from build123d import *

# Parameters (mm, degrees)
BOSS_EXTRUDE1_DEPTH = 25
CUT_EXTRUDE1_DEPTH  = 23
BOSS_EXTRUDE2_DEPTH = 25
BOSS_EXTRUDE3_DEPTH = 2
SKETCH6_R           = 4
BOSS_EXTRUDE4_DEPTH = 10
SKETCH7_R           = 2
CUT_EXTRUDE2_DEPTH  = 54
SKETCH8_R           = 3.5
CUT_EXTRUDE3_DEPTH  = 10
BOSS_EXTRUDE5_DEPTH = 1
FILLET1_R           = 1
SKETCH11_W          = 25
SKETCH11_H          = 84.5
BOSS_EXTRUDE7_DEPTH = 22
CUT_EXTRUDE4_DEPTH  = 34.548411539
SKETCH13_W          = 8.2
SKETCH13_H          = 0.499092091
CUT_EXTRUDE5_DEPTH  = 94.548411539
SKETCH14_W          = 54
SKETCH14_H          = 88
SKETCH14_W_2        = 48
SKETCH14_H_2        = 82.5
CUT_EXTRUDE6_DEPTH  = 1
CUT_EXTRUDE7_DEPTH  = 2
SKETCH16_W          = 8
SKETCH16_H          = 6
CUT_EXTRUDE9_DEPTH  = 2
SKETCH17_W          = 18
SKETCH17_H          = 32
BOSS_EXTRUDE8_DEPTH = 4
SKETCH18_W          = 1.390332564
SKETCH18_H          = 32
BOSS_EXTRUDE9_DEPTH = 3
SKETCH19_W          = 9
SKETCH19_H          = 3.2
CUT_EXTRUDE10_DEPTH = 6
FILLET2_R           = 1
FILLET3_R           = 1
FILLET4_R           = 1
FILLET5_R           = 1
CUT_EXTRUDE12_DEPTH = 1


with BuildPart() as part:
    # Sketch1 → Boss-Extrude1 (new body)
    with BuildSketch(Plane(origin=(0, 0, 0), x_dir=(1, 0, 0), z_dir=(0, 1, 0))):
        with BuildLine():
            Line((-80, 62), (80, 62))
            ThreePointArc((80, 62), (101.213203436, 53.213203436), (110, 32))
            Line((110, 32), (110, -32))
            ThreePointArc((110, -32), (101.213203436, -53.213203436), (80, -62))
            Line((80, -62), (-80, -62))
            ThreePointArc((-80, -62), (-101.213203436, -53.213203436), (-110, -32))
            Line((-110, -32), (-110, 32))
            ThreePointArc((-110, 32), (-101.213203436, 53.213203436), (-80, 62))
        make_face()
    extrude(amount=BOSS_EXTRUDE1_DEPTH)

    # Sketch2 → Cut-Extrude1 (cut)
    with BuildSketch(Plane(origin=(0, 25, 0), x_dir=(1, 0, 0), z_dir=(0, 1, 0))):
        with BuildLine():
            Line((-80, -60), (80, -60))
            ThreePointArc((80, -60), (99.798989873, -51.798989873), (108, -32))
            Line((108, -32), (108, 32))
            ThreePointArc((108, 32), (99.798989873, 51.798989873), (80, 60))
            Line((80, 60), (-80, 60))
            ThreePointArc((-80, 60), (-99.798989873, 51.798989873), (-108, 32))
            Line((-108, 32), (-108, -32))
            ThreePointArc((-108, -32), (-99.798989873, -51.798989873), (-80, -60))
        make_face()
    extrude(amount=-CUT_EXTRUDE1_DEPTH, mode=Mode.SUBTRACT)

    # Sketch3 → Boss-Extrude2 (add)
    with BuildSketch(Plane(origin=(0, 2, 0), x_dir=(1, 0, 0), z_dir=(0, 1, 0))):
        with BuildLine():
            Line((-80, -60), (80, -60))
            ThreePointArc((80, -60), (99.798989873, -51.798989873), (108, -32))
            Line((108, -32), (108, 32))
            ThreePointArc((108, 32), (99.798989873, 51.798989873), (80, 60))
            Line((80, 60), (-80, 60))
            ThreePointArc((-80, 60), (-99.798989873, 51.798989873), (-108, 32))
            Line((-108, 32), (-108, -32))
            ThreePointArc((-108, -32), (-99.798989873, -51.798989873), (-80, -60))
        make_face()
        with BuildLine():
            Line((-80, -59), (80, -59))
            ThreePointArc((80, -59), (99.091883092, -51.091883092), (107, -32))
            Line((107, -32), (107, 32))
            ThreePointArc((107, 32), (99.091883092, 51.091883092), (80, 59))
            Line((80, 59), (-80, 59))
            ThreePointArc((-80, 59), (-99.091883092, 51.091883092), (-107, 32))
            Line((-107, 32), (-107, -32))
            ThreePointArc((-107, -32), (-99.091883092, -51.091883092), (-80, -59))
        make_face(mode=Mode.SUBTRACT)
    extrude(amount=BOSS_EXTRUDE2_DEPTH)

    # Sketch5 → Boss-Extrude3 (add)
    with BuildSketch(Plane.XZ):
        with BuildLine():
            Line((-88, 32), (-88, 20))
            Line((-88, 20), (-90, 20))
            Line((-90, 20), (-90, 32))
            ThreePointArc((-90, 32), (-87.071067812, 39.071067812), (-80, 42))
            Line((-80, 42), (-68, 42))
            Line((-68, 42), (-68, 40))
            Line((-68, 40), (-80, 40))
            ThreePointArc((-80, 40), (-85.656854249, 37.656854249), (-88, 32))
        make_face()
        with BuildLine():
            Line((-80, -40), (-68, -40))
            Line((-68, -40), (-68, -42))
            Line((-68, -42), (-80, -42))
            ThreePointArc((-80, -42), (-87.071067812, -39.071067812), (-90, -32))
            Line((-90, -32), (-90, -20))
            Line((-90, -20), (-88, -20))
            Line((-88, -20), (-88, -32))
            ThreePointArc((-88, -32), (-85.656854249, -37.656854249), (-80, -40))
        make_face()
        with BuildLine():
            Line((88, -32), (88, -20))
            Line((88, -20), (90, -20))
            Line((90, -20), (90, -32))
            ThreePointArc((90, -32), (87.071067812, -39.071067812), (80, -42))
            Line((80, -42), (68, -42))
            Line((68, -42), (68, -40))
            Line((68, -40), (80, -40))
            ThreePointArc((80, -40), (85.656854249, -37.656854249), (88, -32))
        make_face()
        with BuildLine():
            Line((80, 40), (68, 40))
            Line((68, 40), (68, 42))
            Line((68, 42), (80, 42))
            ThreePointArc((80, 42), (87.071067812, 39.071067812), (90, 32))
            Line((90, 32), (90, 20))
            Line((90, 20), (88, 20))
            Line((88, 20), (88, 32))
            ThreePointArc((88, 32), (85.656854249, 37.656854249), (80, 40))
        make_face()
    extrude(amount=BOSS_EXTRUDE3_DEPTH)

    # Sketch6 → Boss-Extrude4 (add)
    with BuildSketch(Plane(origin=(0, 2, 0), x_dir=(1, 0, 0), z_dir=(0, 1, 0))):
        with Locations((80, 32)):
            Circle(SKETCH6_R)
        with Locations((80, -32)):
            Circle(SKETCH6_R)
        with Locations((-80, -32)):
            Circle(SKETCH6_R)
        with Locations((-80, 32)):
            Circle(SKETCH6_R)
    extrude(amount=BOSS_EXTRUDE4_DEPTH)

    # Sketch7 → Cut-Extrude2 (cut)
    with BuildSketch(Plane(origin=(0, 12, 0), x_dir=(1, 0, 0), z_dir=(0, 1, 0))):
        with Locations((80, 32)):
            Circle(SKETCH7_R)
        with Locations((80, -32)):
            Circle(SKETCH7_R)
        with Locations((-80, -32)):
            Circle(SKETCH7_R)
        with Locations((-80, 32)):
            Circle(SKETCH7_R)
    extrude(amount=-CUT_EXTRUDE2_DEPTH, mode=Mode.SUBTRACT)

    # Sketch8 → Cut-Extrude3 (cut)
    with BuildSketch(Plane.XZ):
        with Locations((-80, 32)):
            Circle(SKETCH8_R)
        with Locations((-80, -32)):
            Circle(SKETCH8_R)
        with Locations((80, -32)):
            Circle(SKETCH8_R)
        with Locations((80, 32)):
            Circle(SKETCH8_R)
    extrude(amount=-CUT_EXTRUDE3_DEPTH, mode=Mode.SUBTRACT)

    # Sketch9 → Boss-Extrude5 (add)
    with BuildSketch(Plane(origin=(0, 2, 0), x_dir=(1, 0, 0), z_dir=(0, 1, 0))):
        Polygon((49, -59), (51, -59), (51, -1), (107, -1), (107, 1), (51, 1), (51, 59), (49, 59), (49, 1), (1, 1), (1, 59), (-1, 59), (-1, 1), (-49, 1), (-49, 59), (-51, 59), (-51, 1), (-107, 1), (-107, -1), (-51, -1), (-51, -59), (-49, -59), (-49, -1), (-1, -1), (-1, -59), (1, -59), (1, -1), (49, -1), align=None)
    extrude(amount=BOSS_EXTRUDE5_DEPTH)

    # Fillet1
    fillet1_edges = [part.edges().sort_by_distance(p)[0] for p in [
        (0, 0, 62),
        (-101.213203436, 0, 53.213203436),
        (-110, 0, 0),
        (-101.213203436, 0, -53.213203436),
        (0, 0, -62),
        (101.213203436, 0, -53.213203436),
        (110, 0, 0),
        (101.213203436, 0, 53.213203436),
    ]]
    fillet(fillet1_edges, radius=FILLET1_R)

    # Sketch11 → Boss-Extrude7 (add)
    with BuildSketch(Plane.XZ):
        with Locations((12.5, 0)):
            Rectangle(SKETCH11_W, SKETCH11_H)
        with Locations((-12.5, 0)):
            Rectangle(SKETCH11_W, SKETCH11_H)
    extrude(amount=-BOSS_EXTRUDE7_DEPTH)

    # Sketch12 → Cut-Extrude4 (cut)
    with BuildSketch(Plane(origin=(0, 22, 0), x_dir=(1, 0, 0), z_dir=(0, 1, 0))):
        Polygon((-24, 41.25), (-24, 40.56), (24, -40.56), (24, 41.25), align=None)
        Polygon((24, -40.56), (-24, 40.56), (-24, -41.25), (24, -41.25), align=None)
    extrude(amount=-CUT_EXTRUDE4_DEPTH, mode=Mode.SUBTRACT)

    # Sketch13 → Cut-Extrude5 (cut)
    with BuildSketch(Plane.XY.offset(42.25)):
        with Locations((11.5, 21.750453955)):
            Rectangle(SKETCH13_W, SKETCH13_H)
        with Locations((-11.5, 21.750453955)):
            Rectangle(SKETCH13_W, SKETCH13_H)
    extrude(amount=-CUT_EXTRUDE5_DEPTH, mode=Mode.SUBTRACT)

    # Sketch14 → Cut-Extrude6 (cut)
    with BuildSketch(Plane.XZ):
        Rectangle(SKETCH14_W, SKETCH14_H)
        Rectangle(SKETCH14_W_2, SKETCH14_H_2, mode=Mode.SUBTRACT)
    extrude(amount=-CUT_EXTRUDE6_DEPTH, mode=Mode.SUBTRACT)

    # Sketch15 → Cut-Extrude7 (cut)
    with BuildSketch(Plane.XZ.offset(-1)):
        Polygon((-4, -42.655755812), (-4, -44), (4, -44), (4, -42.655755812), (0, -42.625), align=None)
    extrude(amount=-CUT_EXTRUDE7_DEPTH, mode=Mode.SUBTRACT)

    # Sketch16 → Cut-Extrude9 (cut)
    with BuildSketch(Plane(origin=(0, 3, 0), x_dir=(1, 0, 0), z_dir=(0, 1, 0))):
        with Locations((0, 47)):
            Rectangle(SKETCH16_W, SKETCH16_H)
    extrude(amount=-CUT_EXTRUDE9_DEPTH, mode=Mode.SUBTRACT)

    # Sketch17 → Boss-Extrude8 (add)
    with BuildSketch(Plane(origin=(0, 2, 0), x_dir=(1, 0, 0), z_dir=(0, 1, 0))):
        with Locations((50, 43)):
            Rectangle(SKETCH17_W, SKETCH17_H)
    extrude(amount=BOSS_EXTRUDE8_DEPTH)

    # Sketch18 → Boss-Extrude9 (add, symmetric)
    with BuildSketch(Plane(origin=(0, 6, 0), x_dir=(1, 0, 0), z_dir=(0, 1, 0))):
        with Locations((40.304833718, 43)):
            Rectangle(SKETCH18_W, SKETCH18_H)
        with Locations((59.695166282, 43)):
            Rectangle(SKETCH18_W, SKETCH18_H)
    extrude(amount=BOSS_EXTRUDE9_DEPTH, both=True)

    # Sketch19 → Cut-Extrude10 (cut)
    with BuildSketch(Plane.XY.offset(-59)):
        with Locations((49.8, 9.35)):
            Rectangle(SKETCH19_W, SKETCH19_H)
    extrude(amount=-CUT_EXTRUDE10_DEPTH, mode=Mode.SUBTRACT)

    # Fillet2
    fillet2_edges = [part.edges().sort_by_distance(p)[0] for p in [
        (54.3, 7.75, -60.5),
    ]]
    fillet(fillet2_edges, radius=FILLET2_R)

    # Fillet3
    fillet3_edges = [part.edges().sort_by_distance(p)[0] for p in [
        (45.3, 7.75, -60.5),
    ]]
    fillet(fillet3_edges, radius=FILLET3_R)

    # Fillet4
    fillet4_edges = [part.edges().sort_by_distance(p)[0] for p in [
        (45.3, 10.95, -60.5),
    ]]
    fillet(fillet4_edges, radius=FILLET4_R)

    # Fillet5
    fillet5_edges = [part.edges().sort_by_distance(p)[0] for p in [
        (54.3, 10.95, -60.5),
    ]]
    fillet(fillet5_edges, radius=FILLET5_R)

    # Sketch20 → Cut-Extrude12 (cut)
    with BuildSketch(Plane(origin=(0, 0, -62), x_dir=(-1, 0, 0), z_dir=(0, 0, -1))):
        with BuildLine():
            Line((-56.249828927, 12.40837238), (-43.350171073, 12.40837238))
            ThreePointArc((-43.350171073, 12.40837238), (-42.289510901, 11.969032552), (-41.850171073, 10.90837238))
            Line((-41.850171073, 10.90837238), (-41.850171073, 7.79162762))
            ThreePointArc((-41.850171073, 7.79162762), (-42.289510901, 6.730967448), (-43.350171073, 6.29162762))
            Line((-43.350171073, 6.29162762), (-56.249828927, 6.29162762))
            ThreePointArc((-56.249828927, 6.29162762), (-57.310489099, 6.730967448), (-57.749828927, 7.79162762))
            Line((-57.749828927, 7.79162762), (-57.749828927, 10.90837238))
            ThreePointArc((-57.749828927, 10.90837238), (-57.310489099, 11.969032552), (-56.249828927, 12.40837238))
        make_face()
    extrude(amount=-CUT_EXTRUDE12_DEPTH, mode=Mode.SUBTRACT)


solid = part.part
The listing builds one solid part. Answer for the finished solid, in the listing's coordinates (mm). A direction names the side the tool comes from. Round coordinates to 2 decimals unless told otherwise and drop trailing zeros. Write each loop counter-clockwise with the first axis right and the second up, starting at its lowest first coordinate (ties: lowest second). Pieces come first, ordered by that corner, then holes. Notation, with made-up numbers: M 59.25,4.25 L 108.25,4.25 A20 cw 108.25,18.25 Z; hole C -17,62 d3. An arc over 180 degrees is marked long. Write each question's results on one line, items separated by ' | '. Start each with the question number.
(1) The part is cut by section C-C, the plane x = 73. Write down the section's boundary in (y, z).
(2) Each of these flat-tipped pins is pushed along its axis until it touches: P1, Ø0.8, axis at y = 0.5, z = 15, coming from the -X side (3 decimals); P2, Ø1.1, axis at y = 2.5, z = 49, coming from the +X side; P3, Ø6, axis at x = -26, z = -15.5, coming from the -Y side; P4, Ø12, axis at x = -14.5, z = -4, coming from the -Y side. Where does it stop, or does it pass through?
(3) Find the intervals of material crossed by line 1 (Z direction, x = 38, y = 2.25); line 2 (X direction, y = 2.75, z = 20); line 3 (Z direction, x = 0, y = 6), in increasing order.
(4) For faces 1 (the flat face through (82, 10, -34)), 2 (the flat face through (0, 12, 41.25)), 3 (the cylindrical face through (99.3, 14.32, -50.88)), determine the directions among +Z, -Z, +X, -X, +Y, -Y from which every point of the face is accessible in a straight line to the end or side of a thin tool.
(5) The part is cut by section A-A, the plane y = 16.5. Write down the section's boundary in (x, z), and give its area (3 significant figures).
(6) Determine the mould class of faces 4 (the cylindrical face through (100.979, 12.832, -53.445)), 5 (the cylindrical face through (80.923, 11.014, -30.226)), 6 (the cylindrical face through (-87.15, -0.99, 38.99)) for opening direction X: +X half, -X half, draft (parallel to the pull), parting line (faces both ways), or undercut.
Worked answers:
1) outline: M -2,-42 L 0,-42 L 0,-61 A1 ccw 1,-62 L 25,-62 L 25,-60 L 27,-60 L 27,-59 L 2,-59 L 2,-1 L 3,-1 L 3,1 L 2,1 L 2,59 L 27,59 L 27,60 L 25,60 L 25,62 L 1,62 A1 ccw 0,61 L 0,42 L -2,42 L -2,40 L 0,40 L 0,-40 L -2,-40 Z
2) P1: stops at x = -109.995 | P2: stops at x = 105.09 | P3: stops at y = 0 | P4: passes through
3) line 1: z = -62 to -59, -1 to 1, 59 to 62 | line 2: x = -110 to -107, -51 to -49, -25 to -24, 24 to 25, 49 to 51, 107 to 110 | line 3: z = -62 to -59, -42.25 to -41.25, 41.25 to 42.25, 59 to 62
4) face 1: -Y | face 2: +Y, -Y | face 3: +Y
5) outline: M -110,-32 A30 ccw -80,-62 L 80,-62 A30 ccw 110,-32 L 110,32 A30 ccw 80,62 L -80,62 A30 ccw -110,32 Z; M -25,-42.25 L 25,-42.25 L 25,42.25 L -25,42.25 Z; hole M -107,-32 A27 ccw -80,-59 L 80,-59 A27 ccw 107,-32 L 107,32 A27 ccw 80,59 L -80,59 A27 ccw -107,32 Z; hole M -24,-41.25 L 24,-41.25 L 24,41.25 L -24,41.25 Z | area: 2,150 mm²
6) face 4: +X half | face 5: undercut | face 6: -X half
